from build123d import *

# Parameters (mm, degrees)
F2_R     = 5
F4_D     = 6
F4_DEPTH = 25.001


with BuildPart() as f1:
    # F0 (on Right) → F1 (revolve)
    with BuildSketch(Plane.YZ):
        Polygon((-12.5, 0), (-11, 0), (-11, 38.8), (-25, 38.8), (-25, 18.8), (-12.5, 18.8), (-12.5, 16.8), (-11.95, 16.8), (-11.95, 15.4), (-12.5, 15.4), (-12.5, 3.4), (-11.95, 3.4), (-11.95, 2), (-12.5, 2), align=None)
    revolve(axis=Axis((0, 0, 19.5372104645), (0, 0, 1)))

    # F2
    f2_edges = [f1.edges().sort_by_distance(p)[0] for p in [
        (0, 25, 38.8),
    ]]
    fillet(f2_edges, radius=F2_R)

    # F4 (through all, one way)
    with BuildSketch(Plane.YZ):
        with Locations((0, 28.8)):
            Circle(F4_D / 2)
    extrude(amount=-F4_DEPTH, mode=Mode.SUBTRACT)


solid = f1.part
Design review of the part built by this model. Coordinates are the model's own, in mm. A direction names the side the tool comes from. Round coordinates to 2 decimals unless told otherwise and drop trailing zeros. Write each loop counter-clockwise with the first axis right and the second up, starting at its lowest first coordinate (ties: lowest second). Pieces come first, ordered by that corner, then holes. Notation, with made-up numbers: (-22, 19.25) -> (13, 19.25) arc R12 ccw to (13, 26.25) -> close; hole circle Ø7 at (81, -22.75). An arc over 180 degrees is marked (long way). One line per item, written item: value. Start each with the question number.
Q1. Tool access review of faces 4 (the face through (-17.69, -0.65, 25.87)), 5 (the face through (3.755, -11.923, 9.316)), 6 (the face through (-10, -5, 0)), 7 (the face through (7.509, -23.846, 26.195)), 8 (the face through (10.08, -6.42, 2.69)): name each direction out of +Z, -Z, +X, -X, +Y, -Y from which nothing blocks a thin tool from reaching the whole face with its end or side.
Q2. Add section D-D (z = 28.8). Give the boundary of the cut face in (x, y), then the cut area to 3 significant figures.
Q3. Add section A-A (y = 0). State how many separate pieces and enclosed holes the cut face has, then the cut area to 3 significant figures.
Q4. Insertion check: P1, Ø3, axis at y = 1, z = 6, coming from the -X side; P2, Ø17.5, axis at x = 0, y = 0, coming from the +Z side; P3, Ø5, axis at x = 19, z = 21.5, coming from the +Y side; P4, Ø4, axis at x = -2, z = 11.5, coming from the +Y side. Each pin has a flat end and moves straight along its axis. Give the tip position at first contact, or say it passes through.
Q5. The part is to be moulded in two halves that separate along Z. For faces 1 (the face through (3.755, -11.923, 0.986)), 2 (the face through (10.08, -6.42, 16.09)), 3 (the face through (11.5, 5.9, 18.8)), say which applies: pulls with the +Z half, pulls with the -Z half, needs draft (parallel to the pull), parting line crosses it, or undercut.
Q6. To check wall thickness, follow probe 1 along Z at (x, y) = (-17, 0); probe 2 along X at (y, z) = (0, 24.5); probe 3 along X at (y, z) = (0, 9). State the ranges of each line that lie inside material, in increasing order.
Q7. Add section C-C (z = 9.5). Give the boundary of the cut face in (x, y).
Response:
1. face 4: -X
1. face 5: -Z
1. face 6: -Z, +X, -X, +Y, -Y
1. face 7: +Z, -Z
1. face 8: none
2. outline: (-24.82, -3) arc R25 ccw (long way) to (-24.82, 3) -> (-10.58, 3) arc R11 cw (long way) to (-10.58, -3) -> close
2. area: 1,500 mm^2
3. separate pieces: 3
3. enclosed holes: 0
3. area: 519 mm^2
4. P1: stops at x = -12.5
4. P2: passes through
4. P3: stops at y = 18.78
4. P4: stops at y = 12.5
5. face 1: needs draft
5. face 2: undercut
5. face 3: pulls with the -Z half
6. probe 1: z = 18.8 to 25.8, 31.8 to 38.8
6. probe 2: x = -25 to -11, 11 to 25
6. probe 3: x = -12.5 to -11, 11 to 12.5
7. outline: circle Ø25 at (0, 0); hole circle Ø22 at (0, 0)
